```python
from build123d import *

# Parameters (mm, degrees)
SKETCH2_W                = 46
SKETCH2_H                = 60
BASE_FLANGE1_DEPTH       = 0.86
EDGE_FLANGE1_DEPTH       = 60
EDGE_FLANGE2_DEPTH       = 46
EDGE_FLANGE3_DEPTH       = 60
EDGE_FLANGE5_START       = 0.762
EDGE_FLANGE5_DEPTH       = 35.238
EDGE_FLANGE6_START       = 0.762
EDGE_FLANGE6_DEPTH       = 35.238
M3_CLEARANCE_HOLE1_D     = 3.4
M3_CLEARANCE_HOLE1_DEPTH = 12
M3_CLEARANCE_HOLE1_TIP   = 1.021463052
SKETCH28_R               = 3.4
CUT_EXTRUDE1_DEPTH       = 10
SKETCH29_R               = 4
CUT_EXTRUDE2_DEPTH       = 10
M2_CLEARANCE_HOLE1_D     = 2.4
M2_CLEARANCE_HOLE1_DEPTH = 12
M2_CLEARANCE_HOLE1_TIP   = 0.721032743
M3_CLEARANCE_HOLE2_D     = 3.4
M3_CLEARANCE_HOLE2_DEPTH = 12
M3_CLEARANCE_HOLE2_TIP   = 1.021463052
M2_CLEARANCE_HOLE2_D     = 2.4
M2_CLEARANCE_HOLE4_D     = 2.4
M2_CLEARANCE_HOLE4_DEPTH = 12
M2_CLEARANCE_HOLE4_TIP   = 0.721032743
CUT_EXTRUDE3_DEPTH       = 10
CUT_EXTRUDE4_DEPTH       = 10
CUT_EXTRUDE5_DEPTH       = 10
CUT_EXTRUDE6_DEPTH       = 10
FILLET1_R                = 1
CUT_EXTRUDE7_DEPTH       = 10


# Read off the part's stored shape, not the designer's step: Edge-Flange5, Edge-Flange6
# Sheet-metal steps are written as plain solids
with BuildPart() as part:
    # Sketch2 → Base-Flange1 (new body)
    with BuildSketch(Plane(origin=(0, 0, 0), x_dir=(1, 0, 0), z_dir=(0, 1, 0))):
        Rectangle(SKETCH2_W, SKETCH2_H)
    extrude(amount=-BASE_FLANGE1_DEPTH)

    # Edge-Flange1 section (across the edge) → Edge-Flange1 (add)
    with BuildSketch(Plane(origin=(-23.762, 0, -30), x_dir=(1, 0, 0), z_dir=(0, 0, 1))):
        with BuildLine():
            Line((-0.86, 0.762), (-0.86, 36))
            Line((-0.86, 36), (0, 36))
            Line((0, 36), (0, 0.762))
            ThreePointArc((0, 0.762), (0.223184633, 0.223184633), (0.762, 0))
            Line((0.762, 0), (0.762, -0.86))
            ThreePointArc((0.762, -0.86), (-0.384927199, -0.384927199), (-0.86, 0.762))
        make_face()
    extrude(amount=EDGE_FLANGE1_DEPTH)

    # Edge-Flange2 section (across the edge) → Edge-Flange2 (add)
    with BuildSketch(Plane(origin=(-23, 0, 30.762), x_dir=(0, 0, -1), z_dir=(1, 0, 0))):
        with BuildLine():
            Line((-0.86, 0.762), (-0.86, 36))
            Line((-0.86, 36), (0, 36))
            Line((0, 36), (0, 0.762))
            ThreePointArc((0, 0.762), (0.223184633, 0.223184633), (0.762, 0))
            Line((0.762, 0), (0.762, -0.86))
            ThreePointArc((0.762, -0.86), (-0.384927199, -0.384927199), (-0.86, 0.762))
        make_face()
    edge_flange2 = extrude(amount=EDGE_FLANGE2_DEPTH)

    # Mirror1: Edge-Flange2 across plane
    add(edge_flange2.mirror(Plane.XY))

    # Edge-Flange3 section (across the edge) → Edge-Flange3 (add)
    with BuildSketch(Plane(origin=(23.762, 0, 30), x_dir=(-1, 0, 0), z_dir=(0, 0, -1))):
        with BuildLine():
            Line((-0.86, 0.762), (-0.86, 36))
            Line((-0.86, 36), (0, 36))
            Line((0, 36), (0, 0.762))
            ThreePointArc((0, 0.762), (0.223184633, 0.223184633), (0.762, 0))
            Line((0.762, 0), (0.762, -0.86))
            ThreePointArc((0.762, -0.86), (-0.384927199, -0.384927199), (-0.86, 0.762))
        make_face()
    extrude(amount=EDGE_FLANGE3_DEPTH)

    # Edge-Flange5 outline → Edge-Flange5 (add)
    with BuildSketch(Plane(origin=(0, 0, 0), x_dir=(1, 0, 0), z_dir=(0, 1, 0)).offset(EDGE_FLANGE5_START)):
        with BuildLine():
            ThreePointArc((-24.622, -31.622), (-24.146927199, -32.768927199), (-23, -33.244))
            Line((-23, -33.244), (-15.762, -33.244))
            Line((-15.762, -33.244), (-15.762, -32.384))
            Line((-15.762, -32.384), (-23, -32.384))
            ThreePointArc((-23, -32.384), (-23.538815367, -32.160815367), (-23.762, -31.622))
            Line((-23.762, -31.622), (-23.762, -30))
            Line((-23.762, -30), (-24.622, -30))
            Line((-24.622, -30), (-24.622, -31.622))
        make_face()
    edge_flange5 = extrude(amount=EDGE_FLANGE5_DEPTH)

    # Mirror2: Edge-Flange5 across plane
    add(edge_flange5.mirror(Plane.XY))

    # Edge-Flange6 outline → Edge-Flange6 (add)
    with BuildSketch(Plane(origin=(0, 0, 0), x_dir=(1, 0, 0), z_dir=(0, 1, 0)).offset(EDGE_FLANGE6_START)):
        with BuildLine():
            Line((15.762, -33.244), (23, -33.244))
            ThreePointArc((23, -33.244), (24.146927199, -32.768927199), (24.622, -31.622))
            Line((24.622, -31.622), (24.622, -30))
            Line((24.622, -30), (23.762, -30))
            Line((23.762, -30), (23.762, -31.622))
            ThreePointArc((23.762, -31.622), (23.538815367, -32.160815367), (23, -32.384))
            Line((23, -32.384), (15.762, -32.384))
            Line((15.762, -32.384), (15.762, -33.244))
        make_face()
    edge_flange6 = extrude(amount=EDGE_FLANGE6_DEPTH)

    # Mirror3: Edge-Flange6 across plane
    add(edge_flange6.mirror(Plane.XY))

    # M3 Clearance Hole1
    with Locations(Plane(origin=(0, 0, 0), x_dir=(1, 0, 0), z_dir=(0, 1, 0))):
        with Locations((-20, -27), (20, -27), (-0.5, 27)):
            Hole(M3_CLEARANCE_HOLE1_D / 2, depth=M3_CLEARANCE_HOLE1_DEPTH)
            with Locations((0, 0, -(M3_CLEARANCE_HOLE1_DEPTH + M3_CLEARANCE_HOLE1_TIP / 2))):  # 118° drill point
                Cone(0, M3_CLEARANCE_HOLE1_D / 2, M3_CLEARANCE_HOLE1_TIP, mode=Mode.SUBTRACT)

    # Sketch28 → Cut-Extrude1 (cut)
    with BuildSketch(Plane.ZY.offset(24.622)):
        with Locations(Location((20.78, 15.86, 0), (0, 0, 270))):
            Circle(SKETCH28_R)
    extrude(amount=-CUT_EXTRUDE1_DEPTH, mode=Mode.SUBTRACT)

    # Sketch29 → Cut-Extrude2 (cut)
    with BuildSketch(Plane.ZY.offset(24.622)):
        with Locations(Location((-3.245, 15.762, 0), (0, 0, 270))):
            Circle(SKETCH29_R)
    extrude(amount=-CUT_EXTRUDE2_DEPTH, mode=Mode.SUBTRACT)

    # M2 Clearance Hole1
    with Locations(Plane(origin=(0, -0.86, 0), x_dir=(-1, 0, 0), z_dir=(0, -1, 0))):
        with Locations((-9.869765706, -24.28), (-9.869765706, -18.042)):
            Hole(M2_CLEARANCE_HOLE1_D / 2, depth=M2_CLEARANCE_HOLE1_DEPTH)
            with Locations((0, 0, -(M2_CLEARANCE_HOLE1_DEPTH + M2_CLEARANCE_HOLE1_TIP / 2))):  # 118° drill point
                Cone(0, M2_CLEARANCE_HOLE1_D / 2, M2_CLEARANCE_HOLE1_TIP, mode=Mode.SUBTRACT)

    # M3 Clearance Hole2
    with Locations(Plane(origin=(0, -0.86, 0), x_dir=(-1, 0, 0), z_dir=(0, -1, 0))):
        with Locations((16.23, -6.172321578), (-19.098, -2.172321578), (-19.098, 15.827678422)):
            Hole(M3_CLEARANCE_HOLE2_D / 2, depth=M3_CLEARANCE_HOLE2_DEPTH)
            with Locations((0, 0, -(M3_CLEARANCE_HOLE2_DEPTH + M3_CLEARANCE_HOLE2_TIP / 2))):  # 118° drill point
                Cone(0, M3_CLEARANCE_HOLE2_D / 2, M3_CLEARANCE_HOLE2_TIP, mode=Mode.SUBTRACT)

    # M2 Clearance Hole2 (through all)
    with Locations(Plane.XY.offset(33.244)):
        with Locations((-19.762, 26), (-19.762, 10.762), (19.762, 26), (19.762, 10.754739314)):
            Hole(M2_CLEARANCE_HOLE2_D / 2)

    # M2 Clearance Hole4
    with Locations(Plane(origin=(0, 0, 30.762), x_dir=(-1, 0, 0), z_dir=(0, 0, -1))):
        with Locations((-0.088, 11.622)):
            Hole(M2_CLEARANCE_HOLE4_D / 2, depth=M2_CLEARANCE_HOLE4_DEPTH)
            with Locations((0, 0, -(M2_CLEARANCE_HOLE4_DEPTH + M2_CLEARANCE_HOLE4_TIP / 2))):  # 118° drill point
                Cone(0, M2_CLEARANCE_HOLE4_D / 2, M2_CLEARANCE_HOLE4_TIP, mode=Mode.SUBTRACT)

    # Sketch40 → Cut-Extrude3 (cut)
    with BuildSketch(Plane(origin=(24.622, 0, 0), x_dir=(0, 0, -1), z_dir=(1, 0, 0))):
        with BuildLine():
            Line((-18.622, 22.762), (18.622, 22.762))
            ThreePointArc((18.622, 22.762), (24.622, 16.762), (18.622, 10.762))
            Line((18.622, 10.762), (-18.622, 10.762))
            ThreePointArc((-18.622, 10.762), (-24.622, 16.762), (-18.622, 22.762))
        make_face()
    extrude(amount=-CUT_EXTRUDE3_DEPTH, mode=Mode.SUBTRACT)

    # Sketch42 → Cut-Extrude4 (cut)
    with BuildSketch(Plane(origin=(0, -0.86, 0), x_dir=(-1, 0, 0), z_dir=(0, -1, 0))):
        Polygon((14.53, -6.172321578), (14.53, -9.623545208), (17.93, -9.623545208), (17.93, -7.872321578), (19.704080783, -7.872321578), (19.704080783, -4.002766759), (14.53, -4.002766759), align=None)
    extrude(amount=-CUT_EXTRUDE4_DEPTH, mode=Mode.SUBTRACT)

    # Sketch41 → Cut-Extrude5 (cut)
    with BuildSketch(Plane.XZ.offset(0.86)):
        Polygon((20.798, 2.172321578), (20.798, 5.793483038), (17.398, 5.793483038), (17.398, 4.094032768), (15.692713332, 4.094032768), (15.692713332, 0.472321578), (20.798, 0.472321578), align=None)
    extrude(amount=-CUT_EXTRUDE5_DEPTH, mode=Mode.SUBTRACT)

    # Sketch43 → Cut-Extrude6 (cut)
    with BuildSketch(Plane(origin=(0, -0.86, 0), x_dir=(-1, 0, 0), z_dir=(0, -1, 0))):
        Polygon((-20.798, 15.827678422), (-20.798, 11.962799488), (-17.398, 11.962799488), (-17.398, 13.726356469), (-15.657296152, 13.726356469), (-15.657296152, 17.527678422), (-20.798, 17.527678422), align=None)
    extrude(amount=-CUT_EXTRUDE6_DEPTH, mode=Mode.SUBTRACT)

    # Fillet1
    fillet1_edges = [part.edges().sort_by_distance(p)[0] for p in [
        (-17.93, -0.43, 7.872321578),
        (17.398, -0.43, 4.094032768),
        (17.398, -0.43, -13.726356469),
    ]]
    fillet(fillet1_edges, radius=FILLET1_R)

    # Sketch44 → Cut-Extrude7 (cut)
    with BuildSketch(Plane.ZY.offset(24.622)):
        Polygon((0.755, 15.762), (0, 36), (-7.245, 36), (-7.245, 15.762), align=None)
    extrude(amount=-CUT_EXTRUDE7_DEPTH, mode=Mode.SUBTRACT)


solid = part.part
```
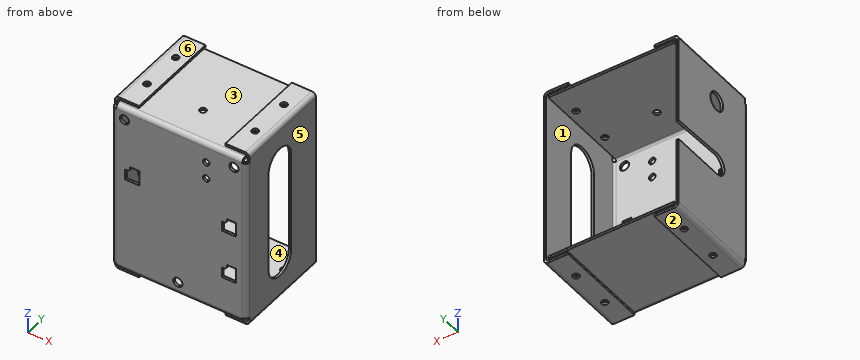
Can you work these out from the model? Positions are in its coordinate system, mm. Face numbers are marked on the shaded views. A direction names the side the tool comes from. Coordinates: 2 decimals unless noted, no trailing zeros. Write each loop counter-clockwise with the first axis right and the second up, starting at its lowest first coordinate (ties: lowest second). Pieces come first, ordered by that corner, then holes. Notation, with made-up numbers: M 32.5,35.5 L 36.5,35.5 A24 ccw 36.5,65.5 Z; hole C -15,7.25 d7. An arc over 180 degrees is marked long. Answer as CSV lines item,"result".
Item 1: On a 3-axis mill with a long thin cutter (end or side, diameter ignored), from which of +Z, -Z, +X, -X, +Y, -Y can I reach the whole of each face in a straight line? I mean the marked faces 1, 2 and 3. Say none if no direction works.
Geometry results:
face 1,"+Y"
face 2,"-Z, +X, -X, +Y, -Y"
face 3,"+Y, -Y"
Item 2: Imagine slicing it at C-C on x = -11. List the corners of the cut face in (y, z) for me.
Geometry results:
outline,"M -0.86,-30 A1.62 ccw 0.76,-31.62 L 36,-31.62 L 36,-30.76 L 0.76,-30.76 A0.76 cw 0,-30 L 0,30 A0.76 cw 0.76,30.76 L 36,30.76 L 36,31.62 L 0.76,31.62 A1.62 ccw -0.86,30 Z"
Item 3: Imagine slicing it at D-D on z = 27. List the corners of the cut face in (x, y) for me, plus the area to 3 significant figures.
Geometry results:
outline,"M -24.62,0.76 A1.62 ccw -23,-0.86 L -21.7,-0.86 L -21.7,0 L -23,0 A0.76 cw -23.76,0.76 L -23.76,36 L -24.62,36 Z; M -18.3,-0.86 L 18.3,-0.86 L 18.3,0 L -18.3,0 Z; M 21.7,-0.86 L 23,-0.86 A1.62 ccw 24.62,0.76 L 24.62,36 L 23.76,36 L 23.76,0.76 A0.76 cw 23,0 L 21.7,0 Z"
area,"97.5 mm2"
Item 4: Imagine slicing it at A-A on z = 2.5. List the corners of the cut face in (x, y) for me.
Geometry results:
outline,"M -24.62,0.76 A1.62 ccw -23,-0.86 L 15.69,-0.86 L 15.69,0 L -23,0 A0.76 cw -23.76,0.76 L -23.76,36 L -24.62,36 Z; M 20.8,-0.86 L 23,-0.86 A1.62 ccw 24.62,0.76 L 24.62,10.76 L 23.76,10.76 L 23.76,0.76 A0.76 cw 23,0 L 20.8,0 Z; M 23.76,22.76 L 24.62,22.76 L 24.62,36 L 23.76,36 Z"
Item 5: I'm going to push flat-ended pins straight in: P1, Ø0.9, axis at x = -18, y = -0.5, coming from the +Z side; P2, Ø10.5, axis at x = 5.5, y = 19, coming from the +Z side; P3, Ø23, axis at x = 1, z = 7, coming from the +Y side. Where does each tip first touch, or does it pass through?
Geometry results:
P1,"stops at z = 31.4"
P2,"stops at z = 31.62"
P3,"stops at y = 0"
Item 6: Please list where these lines run through material, in increasing order: line 1 along Z through (x, y) = (21, 21); line 2 along Z through (x, y) = (8, 26.5); line 3 along X through (y, z) = (34.5, -23.5).
Geometry results:
line 1,"z = -33.24 to -32.38, -31.62 to -30.76, 30.76 to 31.62, 32.38 to 33.24"
line 2,"z = -31.62 to -30.76, 30.76 to 31.62"
line 3,"x = -24.62 to -23.76, 23.76 to 24.62"
Item 7: We'd pull the mould along X, two halves only. Please class the marked faces 4, 5 and 6: +X half, -X half, draft (parallel to the pull), parting line (faces both ways), or undercut.
Geometry results:
face 4,"undercut"
face 5,"+X half"
face 6,"draft"
Item 8: Imagine slicing it at B-B on z = 11.5. List the corners of the cut face in (x, y) for me, plus the area to 3 significant figures.
Geometry results:
outline,"M -24.62,0.76 A1.62 ccw -23,-0.86 L 23,-0.86 A1.62 ccw 24.62,0.76 L 24.62,10.76 L 23.76,10.76 L 23.76,0.76 A0.76 cw 23,0 L -23,0 A0.76 cw -23.76,0.76 L -23.76,36 L -24.62,36 Z; M 23.76,22.76 L 24.62,22.76 L 24.62,36 L 23.76,36 Z"
area,"93.1 mm2"
